Verification items for the finished model (mm, model axes). Face numbers are marked on the shaded views. A direction names the side the tool comes from. Give positions to 0.01 mm unless a question says otherwise; leave off trailing zeros. Order: outer loops, then holes, each group sorted by start corner. A loop starts at its lowest first (then second) coordinate and runs counter-clockwise, first axis right, second up.
(1) Scan lines: L1, parallel to Z at x = 0, y = 164; L2, parallel to Y at x = 12, z = -20.5; L3, parallel to Z at x = 0, y = 278.5. Record each from-to range of solid material in increasing order.
(2) Sectioned sample at A-A on y = 47.5. Record the cut outline in (x, z), plus the area to 3 significant figures.
(3) Access from +Z, -Z, +X, -X, +Y, -Y to the whole of each face (thin tool, end or side, straight path). Record for the marked faces 4 and 5.
(4) Sectioned sample at B-B on z = -24. Record the cut outline in (x, y), plus the area to 3 significant figures.
(5) Mould release check, pull along X, two halves, no side actions. Record for the marked faces 1, 2 and 3: pulls with the +X half, pulls with the -X half, needs draft (parallel to the pull), parting line crosses it, or undercut.
(6) Gauge pin test, flat ends, axial feed: pin 1 (10 mm diameter, centred on x = -37.5, y = 43, fed in from -Z); pin 2 (3 mm diameter, centred on y = 59.5, z = -48, fed in from +X); pin 3 (4 mm diameter, centred on y = 26.5, z = 12.5, fed in from +X). Record the tip position at first contact, or that the pin passes through.
(7) Sectioned sample at D-D on x = -7.5. Record the cut outline in (y, z).
(8) Sectioned sample at C-C on x = -37.5. Record the cut outline in (y, z).
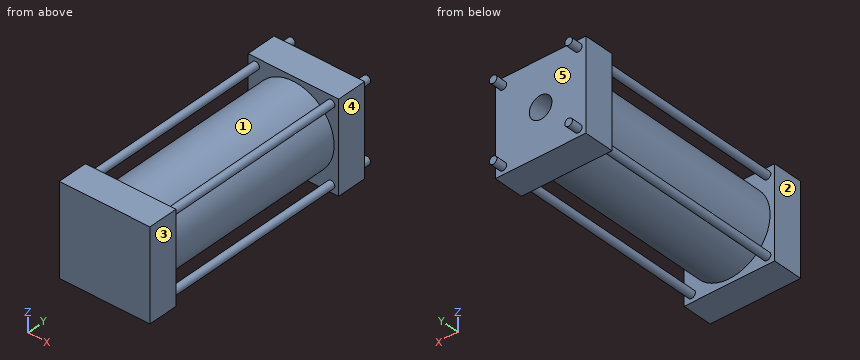
```python
from build123d import *

# Parameters (mm, degrees)
SKETCH1_R            = 54
SKETCH1_R_2          = 50
BOSS_EXTRUDE1_DEPTH  = 250
SKETCH2_W            = 120
SKETCH2_H            = 120
BOSS_EXTRUDE2_DEPTH  = 40
SKETCH3_W            = 120
SKETCH3_H            = 120
BOSS_EXTRUDE3_DEPTH  = 40
CUT_EXTRUDE1_REACH   = 332
SKETCH4_R            = 15
BOSS_EXTRUDE4_START  = -295
SKETCH5_R            = 5
BOSS_EXTRUDE4_DEPTH  = 310
LPATTERN1_COUNT      = 2
LPATTERN1_PITCH      = 100
LPATTERN1_COUNT_DIR2 = 2
LPATTERN1_PITCH_DIR2 = 100


with BuildPart() as part:
    # Sketch1 → Boss-Extrude1 (new body)
    with BuildSketch(Plane(origin=(0, 0, 0), x_dir=(1, 0, 0), z_dir=(0, 1, 0))):
        Circle(SKETCH1_R)
        Circle(SKETCH1_R_2, mode=Mode.SUBTRACT)
    extrude(amount=BOSS_EXTRUDE1_DEPTH)

    # Sketch2 → Boss-Extrude2 (add)
    with BuildSketch(Plane.XZ):
        Rectangle(SKETCH2_W, SKETCH2_H)
    extrude(amount=BOSS_EXTRUDE2_DEPTH)

    # Sketch3 → Boss-Extrude3 (add)
    with BuildSketch(Plane(origin=(0, 250, 0), x_dir=(1, 0, 0), z_dir=(0, 1, 0))):
        Rectangle(SKETCH3_W, SKETCH3_H)
    extrude(amount=BOSS_EXTRUDE3_DEPTH)

    # Sketch4 → Cut-Extrude1 (cut, up to next)
    with BuildSketch(Plane(origin=(0, 290, 0), x_dir=(1, 0, 0), z_dir=(0, 1, 0)), mode=Mode.PRIVATE) as cut_extrude1_sk1:
        Circle(SKETCH4_R)
    cut_extrude1_tool1 = extrude(cut_extrude1_sk1.sketch, amount=-CUT_EXTRUDE1_REACH, mode=Mode.PRIVATE) & part.part
    add(cut_extrude1_tool1.solids().sort_by_distance((0, 290, 0))[0], mode=Mode.SUBTRACT)

    # Sketch5 → Boss-Extrude4 (add)
    with BuildSketch(Plane(origin=(0, 290, 0), x_dir=(1, 0, 0), z_dir=(0, 1, 0)).offset(BOSS_EXTRUDE4_START)):
        with Locations((-50, 50)):
            Circle(SKETCH5_R)
    boss_extrude4 = extrude(amount=BOSS_EXTRUDE4_DEPTH)

    # LPattern1: Boss-Extrude4 2 × 2
    with Locations(*[(i * LPATTERN1_PITCH, 0, j * LPATTERN1_PITCH_DIR2) for i in range(LPATTERN1_COUNT) for j in range(LPATTERN1_COUNT_DIR2) if (i, j) != (0, 0)]):
        add(boss_extrude4)


solid = part.part
```
Ans:
1. L1: z = -54 to -50, 50 to 54
1. L2: y = -40 to 0, 250 to 290
1. L3: z = -60 to -15, 15 to 60
2. outline: circle Ø10 at (-50, -50); circle Ø10 at (-50, 50); circle Ø108 at (0, 0); circle Ø10 at (50, -50); circle Ø10 at (50, 50); hole circle Ø100 at (0, 0)
2. area: 1,620 mm2
3. face 4: +Z, -Z, +X, +Y, -Y
3. face 5: +Y
4. outline: (-60, -40) - (60, -40) - (60, 0) - (48.37, 0) - (48.37, 250) - (60, 250) - (60, 290) - (-60, 290) - (-60, 250) - (-48.37, 250) - (-48.37, 0) - (-60, 0) - close; hole (-43.86, 0) - (43.86, 0) - (43.86, 250) - (-43.86, 250) - close
4. area: 11,900 mm2
5. face 1: undercut
5. face 2: pulls with the -X half
5. face 3: pulls with the +X half
6. pin 1: stops at z = -43.12
6. pin 2: stops at x = 54.97
6. pin 3: stops at x = 52.97
7. outline: (-40, -60) - (0, -60) - (0, -53.48) - (250, -53.48) - (250, -60) - (290, -60) - (290, -12.99) - (250, -12.99) - (250, -49.43) - (0, -49.43) - (0, 49.43) - (250, 49.43) - (250, 12.99) - (290, 12.99) - (290, 60) - (250, 60) - (250, 53.48) - (0, 53.48) - (0, 60) - (-40, 60) - close
8. outline: (-40, -60) - (0, -60) - (0, -38.86) - (250, -38.86) - (250, -60) - (290, -60) - (290, 60) - (250, 60) - (250, 38.86) - (0, 38.86) - (0, 60) - (-40, 60) - close; hole (0, -33.07) - (250, -33.07) - (250, 33.07) - (0, 33.07) - close
